Design review of the part built by this model. Coordinates are the model's own, in mm. Round coordinates to 2 decimals unless told otherwise and drop trailing zeros. Write each loop counter-clockwise with the first axis right and the second up, starting at its lowest first coordinate (ties: lowest second). Pieces come first, ordered by that corner, then holes. Notation, with made-up numbers: M 9,80.5 L 41,80.5 A4 cw 41,86.5 Z; hole C 48.5,39 d1. An arc over 180 degrees is marked long. One line per question, with ' | ' between items. Start each with the question number.
Item 1: Add section C-C, the plane y = -55. State the section outline as (x, z) points, and give its area (3 significant figures).
Item 2: Add section B-B, the plane z = -5.75. State the section outline as (x, y) points.
Item 3: Add section A-A, the plane x = -25. State the section outline as (y, z) points.
Item 4: For L1, parallel to Y at x = 25, z = -7; L2, parallel to Y at x = -21.5, z = -3.25; L3, parallel to X at y = -60, z = -2, list the stretches that pass through material, from the lowest coordinate up.
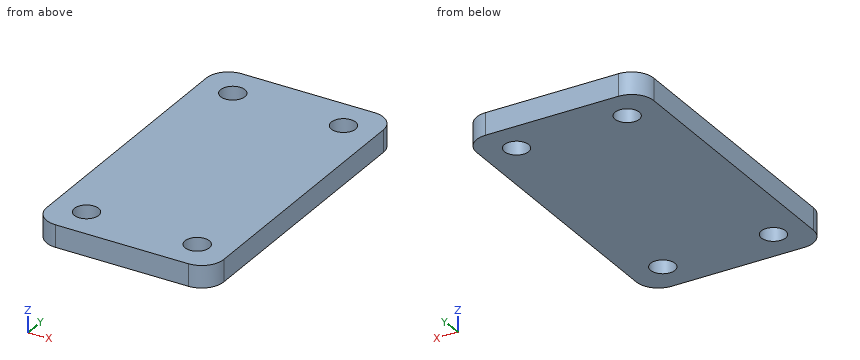
```python
from build123d import *

# Parameters (mm, degrees)
IZIM1_W               = 80
IZIM1_H               = 140
TABAN_FLAN_1_DEPTH    = 10
RADYUS1_R             = 10
IZIM2_R               = 5.5
KES_EKSTR_ZYON1_DEPTH = 20


# Sheet-metal steps are written as plain solids
with BuildPart() as part:
    # Çizim1 → Taban-Flanş1 (new body)
    with BuildSketch(Plane.XY):
        Rectangle(IZIM1_W, IZIM1_H)
    extrude(amount=-TABAN_FLAN_1_DEPTH)

    # Radyus1
    radyus1_edges = [part.edges().sort_by_distance(p)[0] for p in [
        (40, -70, -5),
        (-40, -70, -5),
        (-40, 70, -5),
        (40, 70, -5),
    ]]
    fillet(radyus1_edges, radius=RADYUS1_R)

    # Çizim2 → Kes-Ekstrüzyon1 (cut)
    with BuildSketch(Plane.XY):
        with Locations((25, 55)):
            Circle(IZIM2_R)
        with Locations((-25, 55)):
            Circle(IZIM2_R)
        with Locations((-25, -55)):
            Circle(IZIM2_R)
        with Locations((25, -55)):
            Circle(IZIM2_R)
    extrude(amount=-KES_EKSTR_ZYON1_DEPTH, mode=Mode.SUBTRACT)


solid = part.part
```
Computed values:
1) outline: M -40,-10 L -30.5,-10 L -30.5,0 L -40,0 Z; M -19.5,-10 L 19.5,-10 L 19.5,0 L -19.5,0 Z; M 30.5,-10 L 40,-10 L 40,0 L 30.5,0 Z | area: 580 mm^2
2) outline: M -40,-60 A10 ccw -30,-70 L 30,-70 A10 ccw 40,-60 L 40,60 A10 ccw 30,70 L -30,70 A10 ccw -40,60 Z; hole C -25,-55 d11; hole C -25,55 d11; hole C 25,-55 d11; hole C 25,55 d11
3) outline: M -70,-10 L -60.5,-10 L -60.5,0 L -70,0 Z; M -49.5,-10 L 49.5,-10 L 49.5,0 L -49.5,0 Z; M 60.5,-10 L 70,-10 L 70,0 L 60.5,0 Z
4) L1: y = -70 to -60.5, -49.5 to 49.5, 60.5 to 70 | L2: y = -70 to -59.24, -50.76 to 50.76, 59.24 to 70 | L3: x = -40 to -27.29, -22.71 to 22.71, 27.29 to 40
